Autodesk Inventor part; units mm, degrees
ref_plane "YZ Plane" through (0, 0, 0) normal (1, 0, 0) x (0, 1, 0)
ref_plane "XZ Plane" through (0, 0, 0) normal (0, 1, 0) x (-1, 0, 0)
ref_plane "XY Plane" through (0, 0, 0) normal (0, 0, 1) x (1, 0, 0)
sketch "Sketch1" plane through (0, 0, 0) normal (0, 1, 0) x (-1, 0, 0)
  line L0 (0, 0) -> (5, 0)
  line L1 (5, 0) -> (5, -10)
  line L2 (5, -10) -> (0, -10)
  line L3 (0, -10) -> (0, 0)
  dimension "d0" = 5
  dimension "d1" = 10
extrude "Extrusion1" add sketch "Sketch1" along normal blind 10
sketch "Sketch2" plane through (0, 0, 0) normal (1, 0, 0) x (0, 0, -1)
  line L0 (10, 10) -> (0, 10)
  line L1 (10, 0) -> (10, 10)
  line L2 (0, 10) -> (10, 10)
  line L3 (10, 10) -> (10, 8)
  line L4 (10, 8) -> (0, 8)
  line L5 (0, 8) -> (0, 10)
  line L6 (0, 8) -> (10, 8)
  line L7 (10, 8) -> (10, 5.5)
  line L8 (10, 5.5) -> (0, 5.5)
  line L9 (0, 5.5) -> (0, 8)
  line L10 (0, 5.5) -> (10, 5.5)
  line L11 (10, 5.5) -> (10, 3.5)
  line L12 (10, 3.5) -> (0, 3.5)
  line L13 (0, 3.5) -> (0, 5.5)
  point P0 (0, 0)
  dimension "d4" = 2
  dimension "d5" = 2.5
  dimension "d6" = 2
extrude "Extrusion2" add sketch "Sketch2" along normal blind 5 contours L1 L4 L5 L0 | L1 L12 L13 L8
sketch "Sketch3" plane through (0, 10, 0) normal (0, 1, 0) x (1, 0, 0)
  line L0 (-5, 10) -> (-5, 0)
  line L1 (-5, 0) -> (-2.5, 0)
  line L2 (-2.5, 0) -> (-2.5, 2)
  line L3 (-2.5, 2) -> (-5, 2)
  line L4 (-5, 2) -> (-5, 0)
  line L5 (0, 10) -> (-5, 10)
  line L6 (-5, 10) -> (-2.5, 10)
  line L7 (-2.5, 10) -> (-2.5, 8)
  line L8 (-2.5, 8) -> (-5, 8)
  line L9 (-5, 8) -> (-5, 10)
  circle A0 centre (-2.5, 2) radius 1
  circle A1 centre (-2.5, 8) radius 1
  point P0 (0, 0)
  dimension "d9" = 2.5
  dimension "d10" = 2
  dimension "d11" = 2.5
  dimension "d12" = 2
  dimension "d13" = 2
  dimension "d14" = 2
extrude "Extrusion3" cut sketch "Sketch3" against normal blind 20 contours A1 L7 L8 | L8 L7 A1 | A0 L2 L3 | L3 L2 A0
sketch "Sketch4" plane through (5, 0, 0) normal (1, 0, 0) x (0, 0, -1)
  line L0 (0, 10) -> (0, 8)
  line L1 (0, 8) -> (10, 8)
  line L2 (0, 10) -> (10, 10)
  line L3 (10, 10) -> (10, 8)
  line L4 (10, 8) -> (0, 8)
  line L5 (0, 8) -> (0, 10)
  point P0 (0, 0)
extrude "Extrusion4" cut sketch "Sketch4" against normal blind 4
properties part number "suport1_pcb_temp"
Check sheet for the modelled part. Datum: model origin and axes. Units: mm. A direction names the side the tool comes from. Give positions to 0.01 mm unless a question says otherwise; leave off trailing zeros. Loops run counter-clockwise (first coordinate to the right, second up) from the corner with the lowest first, then second, coordinate; pieces in that order, holes last. Notation, with made-up numbers: M 6,-33 L 34,-33 A34 cw 34,1 Z; hole C 22.25,-28 d6. An arc over 180 degrees is marked long. Answer as a JSON object with one key per item and string values. Group by question number.
Q1. Access from +Z, -Z, +X, -X, +Y, -Y to the whole of each face (thin tool, end or side, straight path). Record for faces 1 (the cylindrical face through (-2.63, 5.07, -8.99)), 2 (the flat face through (0, 2, -5)), 3 (the flat face through (0.5, 8, -5.1)).
Q2. Cross-section at A-A on y = 8.5. Record the cut outline in (x, z).
Q3. Cross-section at C-C on z = -2. Record the cut outline in (x, y), then the cut area to 3 significant figures.
Q4. Go/stop test with flat-tipped pins: P1, Ø4, axis at x = 3.5, z = -7, coming from the -Y side; P2, Ø2, axis at y = 8, z = -3, coming from the +X side; P3, Ø1.8, axis at y = 1.5, z = -3, coming from the +X side. Record where each tip stops, or that it passes through.
Q5. Release check for a two-part mould opening along X. For faces 4 (the cylindrical face through (-2.717, 5.07, -1.024)), 5 (the flat face through (2, 5.5, -5)), 6 (the flat face through (1, 9, -5)) record: released by +X, released by -X, zero draft, split by the parting line, or undercut.
Q6. Cross-section at B-B on x = -2.5. Record the cut outline in (y, z), then the cut area to 3 significant figures.
Q7. Material ranges on line 1 along Z through (x, y) = (-2.5, 4.75); line 2 along X through (y, z) = (4, -2); line 3 along X through (y, z) = (3.25, -8), recorded low to high. Write a range as [from, to].
Q8. Cross-section at D-D on z = -4.25. Record the cut outline in (x, y), then the cut area to 3 significant figures.
Evaluation:
{
 "1": {"face 1": "+Y, -Y", "face 2": "+Z, -Z, +X, -Y", "face 3": "+Z, -Z, +X"},
 "2": {"outline": "M -5,-10 L 1,-10 L 1,0 L -5,0 Z; hole C -2.5,-8 d2; hole C -2.5,-2 d2"},
 "3": {"outline": "M -5,0 L -3.5,0 L -3.5,10 L -5,10 Z; M -1.5,0 L 0,0 L 0,3.5 L 5,3.5 L 5,5.5 L 0,5.5 L 0,8 L 1,8 L 1,10 L -1.5,10 Z", "area": "42.0 mm2"},
 "4": {"P1": "stops at y = 3.5", "P2": "stops at x = 1", "P3": "stops at x = 0"},
 "5": {"face 4": "undercut", "face 5": "zero draft", "face 6": "released by +X"},
 "6": {"outline": "M 0,-10 L 10,-10 L 10,-9 L 0,-9 Z; M 0,-7 L 10,-7 L 10,-3 L 0,-3 Z; M 0,-1 L 10,-1 L 10,0 L 0,0 Z", "area": "60.0 mm2"},
 "7": {"line 1": "z = [-10, -9], [-7, -3], [-1, 0]", "line 2": "x = [-5, -3.5], [-1.5, 5]", "line 3": "x = [-5, -3.5], [-1.5, 0]"},
 "8": {"outline": "M -5,0 L 0,0 L 0,3.5 L 5,3.5 L 5,5.5 L 0,5.5 L 0,8 L 1,8 L 1,10 L -5,10 Z", "area": "62.0 mm2"}
}
